For this review, take the finished solid that the model builds, in its own axes (mm). Coordinates: 2 decimals unless noted, no trailing zeros. Loops run counter-clockwise (first coordinate to the right, second up) from the corner with the lowest first, then second, coordinate; pieces in that order, holes last.
1. Clearance check with a flat-ended pin moving along its axis: P1, Ø2.5, axis at x = 5, y = 135, coming from the -Z side. State where the tip first meets the part, or that it passes through.
2. Take a section at C-C, the plane y = 37.5. State the section outline as (x, z) points.
3. To check wall thickness, follow probe 1 along Y at (x, z) = (5, 0.7); probe 2 along X at (y, z) = (135, 1.3); probe 3 along Y at (x, z) = (6, 1.35). State the ranges of each line that lie inside material, in increasing order.
4. Mouldability with a two-part tool opening along Y and no side actions: class faces 1 (the face through (5, 71, 2)), 2 (the face through (5.9, 38.7, 1)) as pulls with the +Y half, pulls with the -Y half, needs draft (parallel to the pull), parting line crosses it, or undercut.
5. Take a section at B-B, the plane z = 0.5. State the section outline as (x, y) points, then the cut area to 3 significant figures.
6. Take a section at A-A, the plane x = 5. State the section outline as (y, z) points, then the cut area to 3 significant figures.
Autodesk Inventor part; units mm, degrees
ref_plane "YZ Plane" through (0, 0, 0) normal (1, 0, 0) x (0, 1, 0)
ref_plane "XZ Plane" through (0, 0, 0) normal (0, 1, 0) x (-1, 0, 0)
ref_plane "XY Plane" through (0, 0, 0) normal (0, 0, 1) x (1, 0, 0)
sketch "スケッチ1" plane through (0, 0, 0) normal (0, 0, 1) x (1, 0, 0)
  line L0 (0, 0) -> (10, 0)
  line L1 (10, 0) -> (10, 140)
  line L2 (10, 140) -> (0, 140)
  line L3 (0, 140) -> (0, 0)
  dimension "d0" = 10
  dimension "d1" = 140
extrude "押し出し1" add sketch "スケッチ1" along normal blind 2
sketch "スケッチ2" plane through (0, 0, 2) normal (0, 0, 1) x (1, 0, 0)
  line L0 (10, 0) -> (10, 140)
  line L1 (0, 0) -> (10, 0)
  line L2 (10, 140) -> (0, 140)
  point P0 (5, 5)
  point P1 (5, 135)
  dimension "d4" = 5
  dimension "d5" = 5
  dimension "d6" = 5
  dimension "d7" = 5
hole "穴1" at (5, 5, 2) at (5, 135, 2) direction (0, 0, -1) diameter 3 end through all
sketch "スケッチ3" plane through (0, 0, 2) normal (0, 0, 1) x (1, 0, 0)
  circle A0 centre (5, 5) radius 1.5
  point P0 (0, 0)
  point P1 (5, 37.5)
  dimension "d15" = 32.5
hole "穴2" at (5, 37.5, 2) direction (0, 0, -1) diameter 3 end through all
properties part number "レール接続"
Results list:
1. P1: passes through
2. outline: (0, 0) - (3.5, 0) - (3.5, 2) - (0, 2) - close; (6.5, 0) - (10, 0) - (10, 2) - (6.5, 2) - close
3. probe 1: y = 0 to 3.5, 6.5 to 36, 39 to 133.5, 136.5 to 140
3. probe 2: x = 0 to 3.5, 6.5 to 10
3. probe 3: y = 0 to 3.88, 6.12 to 36.38, 38.62 to 133.88, 136.12 to 140
4. face 1: needs draft
4. face 2: undercut
5. outline: (0, 0) - (10, 0) - (10, 140) - (0, 140) - close; hole circle Ø3 at (5, 5); hole circle Ø3 at (5, 37.5); hole circle Ø3 at (5, 135)
5. area: 1,380 mm2
6. outline: (0, 0) - (3.5, 0) - (3.5, 2) - (0, 2) - close; (6.5, 0) - (36, 0) - (36, 2) - (6.5, 2) - close; (39, 0) - (133.5, 0) - (133.5, 2) - (39, 2) - close; (136.5, 0) - (140, 0) - (140, 2) - (136.5, 2) - close
6. area: 262 mm2
